Could you check a few things on this model? Use its own coordinates, in mm. Face numbers are marked on the shaded views. A direction names the side the tool comes from. Give positions to 0.01 mm unless a question says otherwise; leave off trailing zeros. Write each loop counter-clockwise with the first axis right and the second up, starting at its lowest first coordinate (ties: lowest second). Pieces come first, ordered by that corner, then holes. Notation, with made-up numbers: M 46.5,-2 L 53.5,-2 A31 cw 53.5,34 Z; hole C 24,63 d6. An arc over 180 degrees is marked long. Use one line per item in the form item = value.
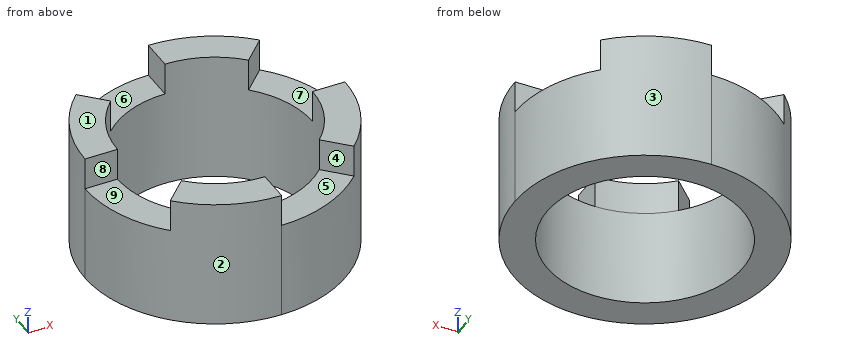
from build123d import *

# Parameters (mm, degrees)
F0_W     = 5.08
F0_H     = 3.175
F1_DEPTH = 25.4
F2_R     = 12.69999
F3_R     = 9.525
F4_DEPTH = 12.701
F6_DEPTH = 3.175


# Not quite as in the source:
# - a fillet or chamfer is up to 0.001 mm smaller than in the source, because OpenCascade refuses the exact size
# - ends of sketch curves that miss each other by under 0.0002 mm in the source are joined


with BuildPart() as f1:
    # F0 (on Front) → F1 (new body)
    with BuildSketch(Plane.XZ):
        Polygon((25.4, 0), (25.4, 12.7), (20.32, 12.7), (20.32, 9.525), (15.24, 9.525), (15.24, 12.7), (10.16, 12.7), (10.16, 9.525), (5.08, 9.525), (5.08, 12.7), (0, 12.7), (0, 0), align=None)
        with Locations((17.78, 11.1125)):
            Rectangle(F0_W, F0_H)
        with Locations((7.62, 11.1125)):
            Rectangle(F0_W, F0_H)
    extrude(amount=F1_DEPTH)

    # F2 (radius 12.7 in the source; OpenCascade refuses exactly that, so slightly less here)
    f2_edges = [f1.edges().sort_by_distance(p)[0] for p in [
        (0, -25.4, 6.35),
        (25.4, -25.4, 6.35),
        (25.4, 0, 6.35),
        (0, 0, 6.35),
    ]]
    fillet(f2_edges, radius=F2_R)

    # F3 (on face) → F4 (cut, through all)
    with BuildSketch(Plane.XY.offset(12.7)):
        with Locations((12.7, -12.7)):
            Circle(F3_R)
    extrude(amount=-F4_DEPTH, mode=Mode.SUBTRACT)

    # F5 (on face) → F6 (cut)
    with BuildSketch(Plane.XY.offset(12.7)):
        with BuildLine():
            ThreePointArc((19.4351920908, -19.4351920908), (21.4999525472, -16.3450596933), (22.225, -12.7))
            ThreePointArc((22.225, -12.7), (21.4999525472, -9.0549403067), (19.4351920908, -5.9648079092))
            ThreePointArc((19.4351920908, -5.9648079092), (16.3450596933, -3.9000474528), (12.7, -3.175))
            ThreePointArc((12.7, -3.175), (9.0549403067, -3.9000474528), (5.9648079092, -5.9648079092))
            ThreePointArc((5.9648079092, -5.9648079092), (3.9000474528, -9.0549403067), (3.175, -12.7))
            ThreePointArc((3.175, -12.7), (3.9000474528, -16.3450596933), (5.9648079092, -19.4351920908))
            ThreePointArc((5.9648079092, -19.4351920908), (9.0549403067, -21.4999525472), (12.7, -22.225))
            ThreePointArc((12.7, -22.225), (16.3450596933, -21.4999525472), (19.4351920908, -19.4351920908))
        make_face()
        with BuildLine():
            ThreePointArc((12.69999, 0), (7.8399142358, -0.9667291759), (3.71974095, -3.71974095))
            Line((3.71974095, -3.71974095), (5.9648079092, -5.9648079092))
            ThreePointArc((5.9648079092, -5.9648079092), (9.0549403067, -3.9000474528), (12.7, -3.175))
            Line((12.7, -3.175), (12.69999, 0))
        make_face()
        with BuildLine():
            ThreePointArc((25.4, -12.69999), (24.4332708241, -7.8399142358), (21.68025905, -3.71974095))
            Line((21.68025905, -3.71974095), (19.4351920908, -5.9648079092))
            ThreePointArc((19.4351920908, -5.9648079092), (21.4999525472, -9.0549403067), (22.225, -12.7))
            Line((22.225, -12.7), (25.4, -12.69999))
        make_face()
        with BuildLine():
            Line((3.175, -12.7), (0, -12.7))
            ThreePointArc((0, -12.7), (0.9667291759, -17.5600857642), (3.71974095, -21.68025905))
            Line((3.71974095, -21.68025905), (5.9648079092, -19.4351920908))
            ThreePointArc((5.9648079092, -19.4351920908), (3.9000474528, -16.3450596933), (3.175, -12.7))
        make_face()
        with BuildLine():
            Line((12.7, -22.225), (12.7, -25.4))
            ThreePointArc((12.7, -25.4), (17.5600857642, -24.4332708241), (21.68025905, -21.68025905))
            Line((21.68025905, -21.68025905), (19.4351920908, -19.4351920908))
            ThreePointArc((19.4351920908, -19.4351920908), (16.3450596933, -21.4999525472), (12.7, -22.225))
        make_face()
    extrude(amount=-F6_DEPTH, mode=Mode.SUBTRACT)


solid = f1.part
1) Thinking about a two-plate mould opening in X: for the marked faces 1, 2, 3 and 4, which applies, released by +X, released by -X, zero draft, split by the parting line, or undercut?
Checked values:
face_1 = zero draft
face_2 = released by -X
face_3 = released by +X
face_4 = undercut
2) I want a section at A-A, the plane z = 10. Count the separate pieces of the cut face and the enclosed holes in it, plus the area to 3 significant figures.
Checked values:
separate_pieces = 4
enclosed_holes = 0
area = 111 mm2
3) For pin 1 Ø1.6 at (x, z) = (2.5, 10.5) entering from -Y; pin 2 Ø2.5 at (y, z) = (-24, 11.5) entering from +X; pin 3 Ø1 at (x, y) = (3, -13.5) entering from +Z (3 decimals), each with a flat end and sliding along its axis, tell me the tip position at first contact or that it passes through.
Checked values:
pin_1 = -12.7
pin_2 = 12.7
pin_3 = 9.525
4) I want a section at D-D, the plane x = 20.5. Please give me the cut outline in (y, z) (3 decimals).
Checked values:
outline = M -22.722,0 L -18.167,0 L -18.167,12.7 L -20.5,12.7 L -20.5,9.525 L -22.722,9.525 Z; M -7.233,0 L -2.678,0 L -2.678,12.7 L -4.9,12.7 L -4.9,9.525 L -7.233,9.525 Z
5) I want a section at B-B, the plane y = -17. Please give me the cut outline in (x, z) (3 decimals).
Checked values:
outline = M 0.75,0 L 4.201,0 L 4.201,9.525 L 0.75,9.525 Z; M 21.199,0 L 24.65,0 L 24.65,12.7 L 21.199,12.7 Z
6) For the marked faces 5, 6, 7, 8 and 9, which set-ups out of +Z, -Z, +X, -X, +Y, -Y let a thin tool reach every point of the face, with its end or its side?
Checked values:
face_5 = +Z, -Y
face_6 = +Z, +Y
face_7 = +Z, +X
face_8 = +Z, -X, -Y
face_9 = +Z, -X
7) If I drill on L1, parallel to Y at x = 12.7, z = 3.25 (3 decimals); L2, parallel to Y at x = 17.75, z = 7.5; L3, parallel to Z at x = 2, y = -19 (3 decimals), over which ranges is the centre line in solid material (lowest first)?
Checked values:
L1 = -25.4 to -22.225, -3.175 to 0
L2 = -24.35 to -20.78, -4.62 to -1.05
L3 = 0 to 9.525
